Model file for the job. Use its own axes, mm. A direction names the side the tool comes from. Round coordinates to 2 decimals unless told otherwise and drop trailing zeros. Loops run counter-clockwise (first coordinate to the right, second up) from the corner with the lowest first, then second, coordinate; pieces in that order, holes last. Notation, with made-up numbers: (44.25, -34) - (100.25, -34) arc R23 cw to (100.25, 1) - close; hole circle Ø6 at (63.5, 62.5). An arc over 180 degrees is marked (long way). Use one line per item in the form item = value.
from build123d import *

# Parameters (mm, degrees)
F0_W     = 4.99
F0_H     = 45
F1_DEPTH = 14.99
F0_W_2   = 10
F2_DEPTH = 10
F0_W_3   = 5
F3_DEPTH = 5
F4_DEPTH = 20
F6_DEPTH = 5
F8_DEPTH = 10
F9_R     = 5


with BuildPart() as f1:
    # F0 (on Top) → F1 (new body)
    with BuildSketch(Plane.XY):
        with Locations((-45.005, 0)):
            Rectangle(F0_W, F0_H)
    extrude(amount=F1_DEPTH)

    # F0 (on Top) → F2 (join)
    with BuildSketch(Plane.XY):
        with Locations((-37.51, 0)):
            Rectangle(F0_W_2, F0_H)
    extrude(amount=F2_DEPTH)

    # F0 (on Top) → F3 (join)
    with BuildSketch(Plane.XY):
        with Locations((-30.01, 0)):
            Rectangle(F0_W_3, F0_H)
    extrude(amount=F3_DEPTH)

    # F0 (on Top) → F4 (join)
    with BuildSketch(Plane.XY):
        Polygon((47.5, 0), (47.5, 22.5), (-27.51, 22.5), (-27.51, -22.5), (47.5, -22.5), align=None)
    extrude(amount=F4_DEPTH)

    # F5 (on face) → F6 (cut)
    with BuildSketch(Plane.XY.offset(20)):
        Polygon((-17.51, -22.5), (2.49, -22.5), (2.49, -17.5), (7.49, -17.5), (7.49, -7.5), (-22.51, -7.5), (-22.51, -12.5), (-22.51, -17.5), (-17.51, -17.5), align=None)
        Polygon((2.49, 17.5), (2.49, 22.5), (-17.51, 22.5), (-17.51, 17.5), (-22.51, 17.5), (-22.51, 7.5), (7.49, 7.5), (7.49, 17.5), align=None)
    extrude(amount=-F6_DEPTH, mode=Mode.SUBTRACT)

    # F7 (on face) → F8 (cut)
    with BuildSketch(Plane.XY):
        Polygon((22.5, -2.5), (27.5, -2.5), (27.5, 0), (27.5, 2.5), (22.5, 2.5), align=None)
    extrude(amount=F8_DEPTH, mode=Mode.SUBTRACT)

    # F9
    f9_edges = [f1.edges().sort_by_distance(p)[0] for p in [
        (47.5, 0, 20),
        (47.5, 22.5, 10),
        (47.5, -22.5, 10),
    ]]
    fillet(f9_edges, radius=F9_R)


solid = f1.part
1. Cut at A-A, the plane z = 6.5. Give the cut face in (x, y).
Geometry check:
outline = (-47.5, -22.5) - (-32.51, -22.5) - (-32.51, 22.5) - (-47.5, 22.5) - close; (-27.51, -22.5) - (42.5, -22.5) arc R5 ccw to (47.5, -17.5) - (47.5, 17.5) arc R5 ccw to (42.5, 22.5) - (-27.51, 22.5) - close; hole (22.5, -2.5) - (27.5, -2.5) - (27.5, 2.5) - (22.5, 2.5) - close
2. Pull direction Y, two halves, no side cores. Call faces 4 (the flat face through (2.49, -20, 18)), 5 (the flat face through (-8, 7.5, 18)), 6 (the flat face through (-3, -22.5, 10)), 7 (the flat face through (8, 22.5, 10)): +Y half, -Y half, draft (parallel to the pull), parting line (faces both ways), or undercut.
Geometry check:
face_4 = draft
face_5 = undercut
face_6 = -Y half
face_7 = +Y half
3. Tool access for faces 1 (the flat face through (-17.51, 20, 18)), 2 (the flat face through (-17.51, -20, 18)), 3 (the flat face through (-22.51, -12, 18)): list every direction of +Z, -Z, +X, -X, +Y, -Y with a clear straight run to the whole face (end or side of a thin tool).
Geometry check:
face_1 = +Z, +Y
face_2 = +Z, -Y
face_3 = +Z
4. Cut at B-B, the plane y = -13.5. Give the cut face in (x, z).
Geometry check:
outline = (-47.5, 0) - (47.5, 0) - (47.5, 15) arc R5 ccw to (42.5, 20) - (7.49, 20) - (7.49, 15) - (-22.51, 15) - (-22.51, 20) - (-27.51, 20) - (-27.51, 5) - (-32.51, 5) - (-32.51, 10) - (-42.51, 10) - (-42.51, 14.99) - (-47.5, 14.99) - close
5. Flat gauge pins, fed straight in: pin 1 (1.5 mm diameter, centred on y = 19, z = 16.5, fed in from -X); pin 2 (1.5 mm diameter, centred on x = -23, y = 6, fed in from -Z); pin 3 (2.5 mm diameter, centred on y = -21, z = 16.5, fed in from +X); pin 4 (2.5 mm diameter, centred on y = -13, z = 17.5, fed in from +X). Where does each tip first touch, or does it go through?
Geometry check:
pin_1 = -27.51
pin_2 = 0
pin_3 = 46.97
pin_4 = 47.34
6. Cut at D-D, the plane x = -3. Give the cut face in (y, z), plus the area to 3 significant figures.
Geometry check:
outline = (-22.5, 0) - (22.5, 0) - (22.5, 15) - (7.5, 15) - (7.5, 20) - (-7.5, 20) - (-7.5, 15) - (-22.5, 15) - close
area = 750 mm^2
7. Cut at C-C, the plane z = 14. Give the cut face in (x, y), plus the area to 3 significant figures.
Geometry check:
outline = (-47.5, -22.5) - (-42.51, -22.5) - (-42.51, 22.5) - (-47.5, 22.5) - close; (-27.51, -22.5) - (42.5, -22.5) arc R5 ccw to (47.5, -17.5) - (47.5, 17.5) arc R5 ccw to (42.5, 22.5) - (-27.51, 22.5) - close
area = 3,590 mm^2
8. Wall check: probe 1 along X at (y, z) = (-4.5, 11.5); probe 2 along Y at (x, z) = (24, 2); probe 3 along X at (y, z) = (13.5, 6). Give the ranges that are in metal, low to high.
Geometry check:
probe_1 = -47.5 to -42.51, -27.51 to 47.5
probe_2 = -22.5 to -2.5, 2.5 to 22.5
probe_3 = -47.5 to -32.51, -27.51 to 47.5
